from build123d import *

# Parameters (mm, degrees)
CUT_EXTRUDE1_START   = -1
CUT_EXTRUDE1_DEPTH   = 5
MIRROR2_START        = -1
MIRROR2_COPY_1_DEPTH = 5
CUT_EXTRUDE2_REACH   = 84.098
SKETCH6_R            = 1.5
CUT_EXTRUDE3_REACH   = 78.968
SKETCH7_R            = 1.5
SKETCH8_R            = 35.200319601
CUT_EXTRUDE4_DEPTH   = 12


with BuildPart() as part:
    # Sweep1: sweep along a path in Sketch1
    with BuildLine(Plane(origin=(0, 0, 0), x_dir=(1, 0, 0), z_dir=(0, 1, 0))) as sweep1_path:
        Line((-28, 62), (28, 62))
        Line((28, 62), (28, 8.339006887))
        ThreePointArc((28, 8.339006887), (28.142356423, 6.017524877), (28.567292497, 3.730830011))
        Line((28.567292497, 3.730830011), (35.074417505, -22.297670018))
        ThreePointArc((35.074417505, -22.297670018), (35.767734257, -26.02859322), (36, -29.816274394))
        Line((36, -29.816274394), (36, -62))
        Line((36, -62), (-36, -62))
        Line((-36, -62), (-36, -29.816274394))
        ThreePointArc((-36, -29.816274394), (-35.767734257, -26.02859322), (-35.074417505, -22.297670018))
        Line((-35.074417505, -22.297670018), (-28.567292497, 3.730830011))
        ThreePointArc((-28.567292497, 3.730830011), (-28.142356423, 6.017524877), (-28, 8.339006887))
        Line((-28, 8.339006887), (-28, 62))
    # Sketch2 → Sweep1 (sweep)
    with BuildSketch(Plane.XY.offset(-62)):
        Polygon((28, 0), (16, 0), (16, 2), (21, 2), (21, 10), (16, 10), (16, 12), (28, 12), (28, 10), (23, 10), (23, 2), (28, 2), align=None)
    sweep(path=sweep1_path.line, transition=Transition.RIGHT)

    # Sweep2: sweep along a path in Sketch3
    with BuildLine(Plane(origin=(28, 0, 0), x_dir=(0, 0, -1), z_dir=(1, 0, 0))) as sweep2_path:
        Line((9, 12), (16.5, 40))
        Line((16.5, 40), (50.5, 40))
        Line((50.5, 40), (58, 12))
    # Sketch4 → Sweep2 (sweep)
    with BuildSketch(Plane(origin=(0, 12, 0), x_dir=(1, 0, 0), z_dir=(0, 1, 0))):
        Polygon((28, 58), (16, 58), (16, 56), (21, 56), (21, 48), (16, 48), (16, 46), (28, 46), (28, 48), (23, 48), (23, 56), (28, 56), align=None)
    sweep2 = sweep(path=sweep2_path.line, transition=Transition.RIGHT)

    # Sketch5 → Cut-Extrude1 (cut)
    with BuildSketch(Plane(origin=(22, 0, 0), x_dir=(0, 0, -1), z_dir=(1, 0, 0)).offset(CUT_EXTRUDE1_START)):
        Polygon((17.661112764, 7.001487652), (18.464285714, 10), (20.464285714, 10), (19.393335317, 6.001785183), align=None)
    cut_extrude1 = extrude(amount=-CUT_EXTRUDE1_DEPTH, mode=Mode.SUBTRACT)

    # Mirror1: Cut-Extrude1 across plane
    add(cut_extrude1.mirror(Plane(origin=(22, 0, 0), x_dir=(0, 0, 1), z_dir=(1, 0, 0))), mode=Mode.SUBTRACT)

    # Mirror2: Sweep2, Cut-Extrude1 across plane
    add(sweep2.mirror(Plane(origin=(0, 0, 0), x_dir=(0, 0, 1), z_dir=(1, 0, 0))))
    add(cut_extrude1.mirror(Plane(origin=(0, 0, 0), x_dir=(0, 0, 1), z_dir=(1, 0, 0))), mode=Mode.SUBTRACT)

    # Mirror2 copy 1 sketch → Mirror2 copy 1 (cut)
    with BuildSketch(Plane(origin=(-22, 0, 0), x_dir=(0, 0, -1), z_dir=(1, 0, 0)).offset(MIRROR2_START)):
        Polygon((17.661112764, 7.001487652), (18.464285714, 10), (20.464285714, 10), (19.393335317, 6.001785183), align=None)
    extrude(amount=-MIRROR2_COPY_1_DEPTH, mode=Mode.SUBTRACT)

    # Sketch6 → Cut-Extrude2 (cut, up to next)
    with BuildSketch(Plane(origin=(0, 40, 0), x_dir=(1, 0, 0), z_dir=(0, 1, 0)), mode=Mode.PRIVATE) as cut_extrude2_sk1:
        with Locations(Location((18.5, 44.5, 0), (0, 0, 180))):
            Circle(SKETCH6_R)
    cut_extrude2_tool1 = extrude(cut_extrude2_sk1.sketch, amount=-CUT_EXTRUDE2_REACH, mode=Mode.PRIVATE) & part.part
    # Sketch6 → Cut-Extrude2 (cut, up to next)
    with BuildSketch(Plane(origin=(0, 40, 0), x_dir=(1, 0, 0), z_dir=(0, 1, 0)), mode=Mode.PRIVATE) as cut_extrude2_sk2:
        with Locations(Location((18.5, 22.5, 0), (0, 0, 180))):
            Circle(SKETCH6_R)
    cut_extrude2_tool2 = extrude(cut_extrude2_sk2.sketch, amount=-CUT_EXTRUDE2_REACH, mode=Mode.PRIVATE) & part.part
    # Sketch6 → Cut-Extrude2 (cut, up to next)
    with BuildSketch(Plane(origin=(0, 40, 0), x_dir=(1, 0, 0), z_dir=(0, 1, 0)), mode=Mode.PRIVATE) as cut_extrude2_sk3:
        with Locations(Location((-18.5, 44.5, 0), (0, 0, 180))):
            Circle(SKETCH6_R)
    cut_extrude2_tool3 = extrude(cut_extrude2_sk3.sketch, amount=-CUT_EXTRUDE2_REACH, mode=Mode.PRIVATE) & part.part
    # Sketch6 → Cut-Extrude2 (cut, up to next)
    with BuildSketch(Plane(origin=(0, 40, 0), x_dir=(1, 0, 0), z_dir=(0, 1, 0)), mode=Mode.PRIVATE) as cut_extrude2_sk4:
        with Locations(Location((-18.5, 22.5, 0), (0, 0, 180))):
            Circle(SKETCH6_R)
    cut_extrude2_tool4 = extrude(cut_extrude2_sk4.sketch, amount=-CUT_EXTRUDE2_REACH, mode=Mode.PRIVATE) & part.part
    add(cut_extrude2_tool1.solids().sort_by_distance((18.5, 40, -44.5))[0], mode=Mode.SUBTRACT)
    add(cut_extrude2_tool2.solids().sort_by_distance((18.5, 40, -22.5))[0], mode=Mode.SUBTRACT)
    add(cut_extrude2_tool3.solids().sort_by_distance((-18.5, 40, -44.5))[0], mode=Mode.SUBTRACT)
    add(cut_extrude2_tool4.solids().sort_by_distance((-18.5, 40, -22.5))[0], mode=Mode.SUBTRACT)

    # Sketch7 → Cut-Extrude3 (cut, up to next)
    with BuildSketch(Plane(origin=(0, 12, 0), x_dir=(1, 0, 0), z_dir=(0, 1, 0)), mode=Mode.PRIVATE) as cut_extrude3_sk1:
        with Locations(Location((33, -32, 0), (0, 0, 270))):
            Circle(SKETCH7_R)
    cut_extrude3_tool1 = extrude(cut_extrude3_sk1.sketch, amount=-CUT_EXTRUDE3_REACH, mode=Mode.PRIVATE) & part.part
    # Sketch7 → Cut-Extrude3 (cut, up to next)
    with BuildSketch(Plane(origin=(0, 12, 0), x_dir=(1, 0, 0), z_dir=(0, 1, 0)), mode=Mode.PRIVATE) as cut_extrude3_sk2:
        with Locations(Location((33, -56, 0), (0, 0, 270))):
            Circle(SKETCH7_R)
    cut_extrude3_tool2 = extrude(cut_extrude3_sk2.sketch, amount=-CUT_EXTRUDE3_REACH, mode=Mode.PRIVATE) & part.part
    # Sketch7 → Cut-Extrude3 (cut, up to next)
    with BuildSketch(Plane(origin=(0, 12, 0), x_dir=(1, 0, 0), z_dir=(0, 1, 0)), mode=Mode.PRIVATE) as cut_extrude3_sk3:
        with Locations((-33, -56)):
            Circle(SKETCH7_R)
    cut_extrude3_tool3 = extrude(cut_extrude3_sk3.sketch, amount=-CUT_EXTRUDE3_REACH, mode=Mode.PRIVATE) & part.part
    # Sketch7 → Cut-Extrude3 (cut, up to next)
    with BuildSketch(Plane(origin=(0, 12, 0), x_dir=(1, 0, 0), z_dir=(0, 1, 0)), mode=Mode.PRIVATE) as cut_extrude3_sk4:
        with Locations((-33, -32)):
            Circle(SKETCH7_R)
    cut_extrude3_tool4 = extrude(cut_extrude3_sk4.sketch, amount=-CUT_EXTRUDE3_REACH, mode=Mode.PRIVATE) & part.part
    add(cut_extrude3_tool1.solids().sort_by_distance((33, 12, 32))[0], mode=Mode.SUBTRACT)
    add(cut_extrude3_tool2.solids().sort_by_distance((33, 12, 56))[0], mode=Mode.SUBTRACT)
    add(cut_extrude3_tool3.solids().sort_by_distance((-33, 12, 56))[0], mode=Mode.SUBTRACT)
    add(cut_extrude3_tool4.solids().sort_by_distance((-33, 12, 32))[0], mode=Mode.SUBTRACT)

    # Sketch8 → Cut-Extrude4 (cut)
    with BuildSketch(Plane.XY.offset(62)):
        with Locations((0, 40.25)):
            Circle(SKETCH8_R)
    extrude(amount=-CUT_EXTRUDE4_DEPTH, mode=Mode.SUBTRACT)


solid = part.part
Model file for the job. Use its own axes, mm. A direction names the side the tool comes from. Give positions to 0.01 mm unless a question says otherwise; leave off trailing zeros. Order: outer loops, then holes, each group sorted by start corner. A loop starts at its lowest first (then second) coordinate and runs counter-clockwise, first axis right, second up. Notation, with made-up numbers: (49, 35.25) - (81, 35.25) arc R31 cw to (81, 63.25) - close; hole circle Ø11 at (60, 46). An arc over 180 degrees is marked (long way). One line per item, written item: value.
Item 1: Pin check, flat tips, straight feed: pin 1 Ø3 at (x, y) = (18.5, 28.5) entering from +Z; pin 2 Ø11 at (x, z) = (5.5, -55.5) entering from +Y; pin 3 Ø24 at (y, z) = (31, -24.5) entering from +X; pin 4 Ø2 at (x, z) = (-28, 22) entering from -Y. Stop position of each tip, or through.
Response values:
pin 1: z = -13.02
pin 2: y = 12
pin 3: x = 28
pin 4: y = 0
Item 2: Two-plate mould, pull along Y, no slides. Class faces 6 (the flat face through (0, 6, -57)), 7 (the flat face through (-31.775, 10.986, 9.101)), 8 (the flat face through (25, 0, 1)), 9 (the flat face through (-22.084, 25.804, -54.303)): released by +Y, released by -Y, zero draft, split by the parting line, or undercut.
Response values:
face 6: undercut
face 7: zero draft
face 8: released by -Y
face 9: released by +Y
Item 3: Slice it at C-C (x = 10.5). List the corners of the cut face in (y, z).
Response values:
outline: (0, -62) - (2, -62) - (2, -57) - (10, -57) - (10, -62) - (12, -62) - (12, -50) - (10, -50) - (10, -55) - (2, -55) - (2, -50) - (0, -50) - close; (0, 50) - (2, 50) - (2, 55) - (6.65, 55) - (6.65, 57) - (2, 57) - (2, 62) - (0, 62) - close
Item 4: Slice it at B-B (x = -33). List the corners of the cut face in (y, z), then the cut area to 3 significant figures.
Response values:
outline: (0, 14) - (2, 14) - (2, 62) - (0, 62) - close; (10, 14) - (12, 14) - (12, 30.5) - (10, 30.5) - close; (10, 33.5) - (12, 33.5) - (12, 54.5) - (10, 54.5) - close; (10, 57.5) - (12, 57.5) - (12, 62) - (10, 62) - close
area: 180 mm2
Item 5: Wall check: line 1 (X direction, y = 10.8, z = 32); line 2 (X direction, y = 36, z = -35.5); line 3 (Z direction, x = -14.5, y = 3). Give the ranges that are in metal, low to high.
Response values:
line 1: -36 to -34.5, -31.5 to -24, 24 to 31.5, 34.5 to 36
line 2: -23 to -21, 21 to 23
line 3: -57 to -55, 55 to 57
Item 6: Slice it at A-A (z = 40). List the corners of the cut face in (x, y).
Response values:
outline: (-36, 0) - (-24, 0) - (-24, 2) - (-29, 2) - (-29, 10) - (-24, 10) - (-24, 12) - (-36, 12) - (-36, 10) - (-31, 10) - (-31, 2) - (-36, 2) - close; (24, 0) - (36, 0) - (36, 2) - (31, 2) - (31, 10) - (36, 10) - (36, 12) - (24, 12) - (24, 10) - (29, 10) - (29, 2) - (24, 2) - close
Item 7: Tool access for faces 1 (the flat face through (26, 30.341, -34)), 2 (the flat face through (-28, 29, -37)), 3 (the flat face through (-17, 2, -4)), 4 (the cylindrical face through (23.175, 6.056, -5.447)), 5 (the flat face through (21.916, 20.089, -43.833)): list every direction of +Z, -Z, +X, -X, +Y, -Y with a clear straight run to the whole face (end or side of a thin tool).
Response values:
face 1: +X
face 2: -Z, -X, +Y, -Y
face 3: none
face 4: -Z, +X
face 5: +X, -X
